Work out the finished part from the listing and answer in its coordinate system (mm). Face numbers are marked on the shaded views. Coordinates: 2 decimals unless noted, no trailing zeros. Write each loop counter-clockwise with the first axis right and the second up, starting at its lowest first coordinate (ties: lowest second). Pieces come first, ordered by that corner, then holes. Notation, with made-up numbers: (-29.75, 12) - (27.25, 12) arc R22 ccw to (27.25, 31) - close; hole circle Ø8 at (11, 48). An arc over 180 degrees is marked (long way). Use one line per item in the form item = value. Start each with the question number.
Item 1: A cutting plane is placed at C-C (z = -2.5). Write down the section's boundary in (x, y), then the cut area to 3 significant figures.
Item 2: Determine the mould class of the marked faces 1, 2 and 3 for opening direction Y: released by +Y, released by -Y, zero draft, split by the parting line, or undercut.
Item 3: A cutting plane is placed at B-B (x = 3.25). Write down the section's boundary in (y, z).
Item 4: A cutting plane is placed at A-A (y = 18.5). Write down the section's boundary in (x, z).
Item 5: Given pin 1 (2 mm diameter, centred on y = 12.5, z = 3, fed in from +X); pin 2 (3 mm diameter, centred on y = 12.5, z = 3, fed in from -X); pin 3 (1 mm diameter, centred on x = 2, y = 13, fed in from -Z), each flat-ended and moving along its own axis, determine where each tip first touches the part or whether it passes through.
Item 6: Consider probe 1 along Y at (x, z) = (0.75, 2); probe 2 along Z at (x, y) = (1, 6.25); probe 3 along Z at (x, y) = (2.75, 19.25). Determine where each line is inside the solid, lowest interval first.
from build123d import *

# Parameters (mm, degrees)
CUT_EXTRUDE_START        = -4.3
CUT_EXTRUDE_1_DEPTH      = 4.3
PATTERN_CIRCULAR_1_COUNT = 11
PATTERN_CIRCULAR_1_ANGLE = 330


with BuildPart() as part:
    # ｽｹｯﾁ1 → 回転1 (revolve)
    with BuildSketch(Plane.XY, mode=Mode.PRIVATE) as revolve_1_sk:
        Polygon((0, 0), (0, 26.1), (1, 26.1), (1, 26), (2, 26), (2, 22), (1, 22), (1, 20), (4, 20), (4, 0), align=None)
    revolve(revolve_1_sk.sketch.rotate(Axis((0, 0, 0), (0, 1, 0)), 90), axis=Axis((0, 0, 0), (0, 1, 0)))

    # ｽｹｯﾁ3 → ｶｯﾄ - 押し出し1 (cut)
    with BuildSketch(Plane(origin=(0, 26, 0), x_dir=(1, 0, 0), z_dir=(0, 1, 0)).offset(CUT_EXTRUDE_START)):
        with BuildLine():
            ThreePointArc((0.092905413, 1.299949383), (0.266119458, 1.637619869), (0.5, 1.936491673))
            ThreePointArc((0.5, 1.936491673), (0, 2), (-0.5, 1.936491673))
            ThreePointArc((-0.5, 1.936491673), (-0.266119458, 1.637619869), (-0.092905413, 1.299949383))
            ThreePointArc((-0.092905413, 1.299949383), (0, 1.236943764), (0.092905413, 1.299949383))
        make_face()
    cut_extrude_1 = extrude(amount=CUT_EXTRUDE_1_DEPTH, mode=Mode.SUBTRACT)

    # 円形ﾊﾟﾀｰﾝ1: ｶｯﾄ - 押し出し1 ×11 about axis
    pattern_circular_1_axis = Axis((0, 0, 0), (0, -1, 0))
    for i in range(1, PATTERN_CIRCULAR_1_COUNT):
        add(cut_extrude_1.rotate(pattern_circular_1_axis, i * PATTERN_CIRCULAR_1_ANGLE / (PATTERN_CIRCULAR_1_COUNT - 1)), mode=Mode.SUBTRACT)


solid = part.part
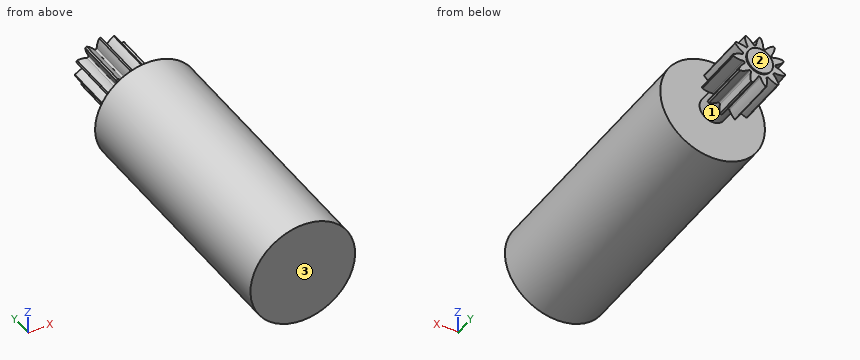
Answer:
q1.outline = (-3.12, 0) - (3.12, 0) - (3.12, 20) - (-3.12, 20) - close
q1.area = 125 mm²
q2.face_1 = undercut
q2.face_2 = released by +Y
q2.face_3 = released by -Y
q3.outline = (0, -2.33) - (20, -2.33) - (20, 2.33) - (0, 2.33) - close
q4.outline = circle Ø8 at (0, 0)
q5.pin_1 = 3.46
q5.pin_2 = -3.71
q5.pin_3 = -3.71
q6.probe_1 = 0 to 20
q6.probe_2 = -3.87 to 3.87
q6.probe_3 = -2.9 to 2.9
